Check sheet for the drawn part. Datum: minimum x, y, z corner. Units: mm. A direction names the side the tool comes from. Round coordinates to 2 decimals unless told otherwise and drop trailing zeros. Write each loop counter-clockwise with the first axis right and the second up, starting at its lowest first coordinate (ties: lowest second). Pieces come first, ordered by that corner, then holes. Notation, with made-up numbers: (7, -20.75) - (34, -20.75) arc R28 ccw to (34, 15.25) - close; hole circle Ø11 at (89, 1). An arc over 180 degrees is marked (long way). Answer as a JSON object with one key per item and string values.
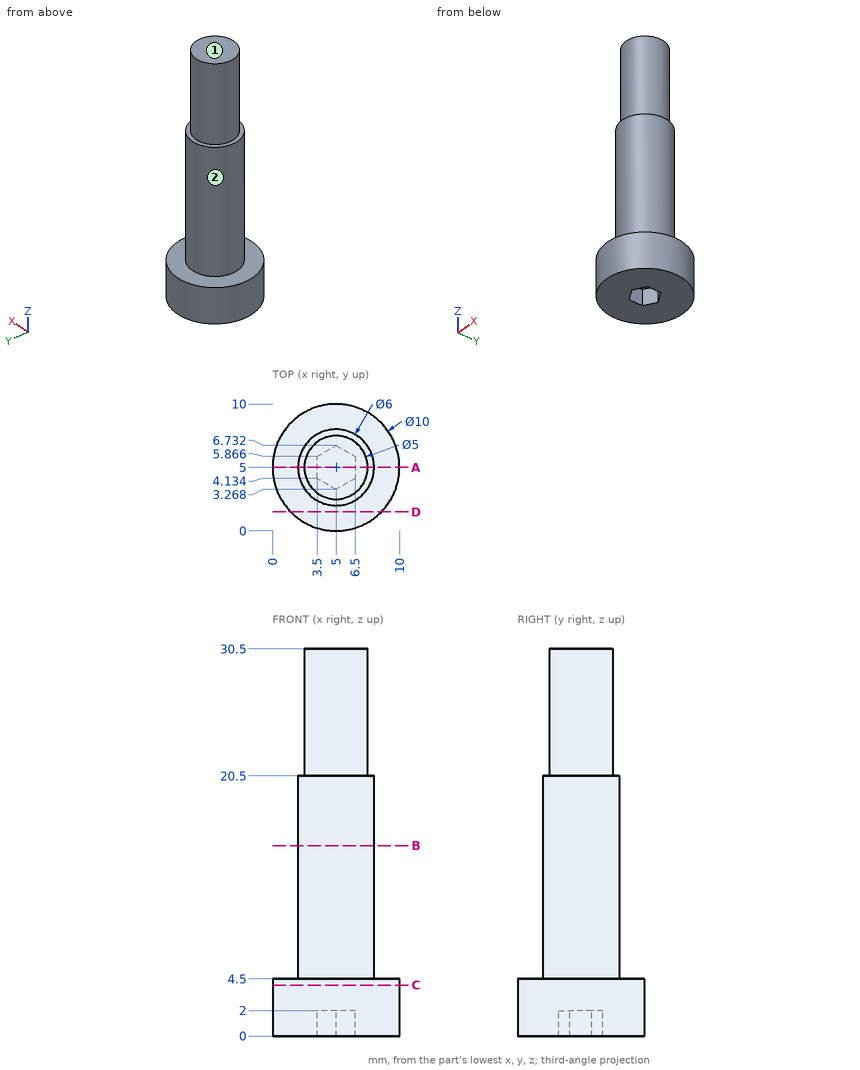
Q1. Section check D-D, the plane y = 1.5. Record the cut outline in (x, z).
Geometry check:
{"outline": "(1.43, 0) - (8.57, 0) - (8.57, 4.5) - (1.43, 4.5) - close"}
Q2. Section check C-C, the plane z = 4. Record the cut outline in (x, y), then the cut area to 3 significant figures.
Geometry check:
{"outline": "circle Ø10 at (5, 5)", "area": "78.5 mm2"}
Q3. Set-up check for the marked faces 1 and 2: record each of +Z, -Z, +X, -X, +Y, -Y from which the full face is reachable in a straight line by a thin tool's end or side.
Geometry check:
{"face 1": "+Z, +X, -X, +Y, -Y", "face 2": "+Z"}
Q4. Section check B-B, the plane z = 15. Record the cut outline in (x, y), then the cut area to 3 significant figures.
Geometry check:
{"outline": "circle Ø6 at (5, 5)", "area": "28.3 mm2"}
Q5. Section check A-A, the plane y = 5. Record the cut outline in (x, z).
Geometry check:
{"outline": "(0, 0) - (3.5, 0) - (3.5, 2) - (6.5, 2) - (6.5, 0) - (10, 0) - (10, 4.5) - (8, 4.5) - (8, 20.5) - (7.5, 20.5) - (7.5, 30.5) - (2.5, 30.5) - (2.5, 20.5) - (2, 20.5) - (2, 4.5) - (0, 4.5) - close"}
Q6. Gauge pin test, flat ends, axial feed: P1, Ø5, axis at y = 4.5, z = 9.5, coming from the -X side; P2, Ø6, axis at y = 8.5, z = 10.5, coming from the +X side; P3, Ø1.5, axis at y = 5, z = 25.5, coming from the -X side. Record the tip position at first contact, or that the pin passes through.
Geometry check:
{"P1": "stops at x = 2", "P2": "stops at x = 7.96", "P3": "stops at x = 2.5"}
Q7. Material ranges on line 1 along Y through (x, z) = (5, 15); line 2 along Y through (x, z) = (5, 22); line 3 along Z through (x, y) = (1.25, 3.5), recorded low to high. Write a range as [from, to].
Geometry check:
{"line 1": "y = [2, 8]", "line 2": "y = [2.5, 7.5]", "line 3": "z = [0, 4.5]"}
